The model under review builds one solid part; all positions refer to its coordinate system, in mm. A direction names the side the tool comes from. Coordinates: 2 decimals unless noted, no trailing zeros. Write each loop counter-clockwise with the first axis right and the second up, starting at its lowest first coordinate (ties: lowest second). Pieces come first, ordered by that corner, then holes. Notation, with made-up numbers: (17, -27) - (69, -27) arc R26 ccw to (69, -11) - close; hole circle Ø7 at (52.25, 47.5). An arc over 180 degrees is marked (long way). Answer as CSV lines item,"result". Start each with the question number.
Autodesk Inventor part; units mm, degrees
ref_plane "YZ Plane" through (0, 0, 0) normal (1, 0, 0) x (0, 1, 0)
ref_plane "XZ Plane" through (0, 0, 0) normal (0, 1, 0) x (-1, 0, 0)
ref_plane "XY Plane" through (0, 0, 0) normal (0, 0, 1) x (1, 0, 0)
sketch "Sketch1" plane through (0, 0, 0) normal (0, 0, 1) x (1, 0, 0)
  line L0 (0, 0) -> (20, 0)
  line L1 (20, 0) -> (20, 3.2)
  line L2 (20, 3.2) -> (0, 3.2)
  line L3 (0, 3.2) -> (0, 0)
  line L4 (20, 0) -> (36.65, 0)
  line L5 (36.65, 0) -> (36.65, 6.335)
  line L6 (36.65, 6.335) -> (20, 6.335)
  line L7 (20, 6.335) -> (20, 0)
  line L8 (36.65, 0) -> (53.17, 0)
  line L9 (53.17, 0) -> (53.17, 7.26)
  line L10 (53.17, 7.26) -> (36.65, 7.26)
  line L11 (36.65, 7.26) -> (36.65, 0)
  line L12 (53.17, 0) -> (102.07, 0)
  line L13 (102.07, 0) -> (102.07, 9)
  line L14 (102.07, 9) -> (64.2031, 9)
  line L15 (53.17, 9) -> (53.17, 0)
  line L16 (102.07, 0) -> (117.1074, 0)
  line L17 (117.1074, 0) -> (117.1074, 4.5)
  line L18 (117.1074, 4.5) -> (102.07, 4.5)
  line L19 (102.07, 4.5) -> (102.07, 0)
  line L20 (53.17, 8.2611) -> (64.2031, 9)
  dimension "d0" = 20
  dimension "d1" = 3.2
  dimension "d2" = 16.65
  dimension "d3" = 6.335
  dimension "d4" = 16.52
  dimension "d5" = 7.26
  dimension "d6" = 48.9
  dimension "d7" = 9
revolve "Revolution1" add sketch "Sketch1" angle 360 about axis through (53.17, 0, 0) along (1, 0, 0)
properties part number "00_Micrometer"
(1) For faces 1 (the flat face through (117.107, 0, 0)), 2 (the cylindrical face through (9.86, -2.539, 1.947)), 3 (the cylindrical face through (109.48, -0.59, -4.46)), list the 3-axis set-ups (+Z, -Z, +X, -X, +Y, -Y) from which the entire face can be reached by the end or side of a thin tool; tool diameter is ignored.
(2) For pin 1 (5 mm diameter, centred on y = 4, z = -6, fed in from -X); pin 2 (3 mm diameter, centred on x = 40.5, y = 4, fed in from +Z); pin 3 (4 mm diameter, centred on x = 99.5, y = 5.5, fed in from +Z), all flat-tipped, find the tip position at first contact; note any pin that passes through.
(3) Add section C-C on x = 35.5. Give the boundary of the cut face in (y, z) (3 decimals), then the cut area to 3 significant figures.
(4) Add section A-A on y = 0. Give the boundary of the cut face in (x, z) (3 decimals), then the cut area to 3 significant figures.
(5) Wall thickness on line 1 (X direction, y = -5, z = -2); line 2 (Y direction, x = 20.5, z = -0.5); line 3 (X direction, y = 7.75, z = 2.75): over which ranges is each line inside the solid? List them lowest first.
(6) Add section D-D on x = 19. Give the boundary of the cut face in (y, z).
Reported:
1,face 1,"+Z, -Z, +X, +Y, -Y"
1,face 2,"-X"
1,face 3,"+X"
2,pin 1,"x = 20"
2,pin 2,"z = 6.82"
2,pin 3,"z = 8.29"
3,outline,"circle Ø12.67 at (0, 0)"
3,area,"126 mm²"
4,outline,"(0, -3.2) - (20, -3.2) - (20, -6.335) - (36.65, -6.335) - (36.65, -7.26) - (53.17, -7.26) - (53.17, -8.261) - (64.203, -9) - (102.07, -9) - (102.07, -4.5) - (117.107, -4.5) - (117.107, 4.5) - (102.07, 4.5) - (102.07, 9) - (64.203, 9) - (53.17, 8.261) - (53.17, 7.26) - (36.65, 7.26) - (36.65, 6.335) - (20, 6.335) - (20, 3.2) - (0, 3.2) - close"
4,area,"1,590 mm²"
5,line 1,"20 to 102.07"
5,line 2,"-6.32 to 6.32"
5,line 3,"53.17 to 102.07"
6,outline,"circle Ø6.4 at (0, 0)"
